```python
from build123d import *

# Parameters (mm, degrees)
BOSS_EXTRUDE1_DEPTH = 6.35
SKETCH2_R           = 3.302
SKETCH2_R_2         = 3.4798
SKETCH2_R_3         = 3.6576
CUT_EXTRUDE1_DEPTH  = 7.35
SHELL5_T            = -2.54
SKETCH5_R           = 6.0198
BOSS_EXTRUDE5_DEPTH = 3.81
SKETCH8_W           = 1.524
SKETCH8_H           = 8.89
CUT_EXTRUDE2_DEPTH  = 6.35
CHAMFER1_SIZE       = 0.635


with BuildPart() as part:
    # Sketch1 → Boss-Extrude1 (new body)
    with BuildSketch(Plane.XY):
        with BuildLine():
            Line((-38.1, 6.35), (38.1, 6.35))
            ThreePointArc((38.1, 6.35), (44.45, 0), (38.1, -6.35))
            Line((38.1, -6.35), (-38.1, -6.35))
            ThreePointArc((-38.1, -6.35), (-44.45, 0), (-38.1, 6.35))
        make_face()
    extrude(amount=BOSS_EXTRUDE1_DEPTH)

    # Sketch2 → Cut-Extrude1 (cut, through all)
    with BuildSketch(Plane.XY.offset(6.35)):
        with Locations((-38.1, 0)):
            Circle(SKETCH2_R)
        with Locations((-12.7, 0)):
            Circle(SKETCH2_R_2)
        with Locations((12.7, 0)):
            Circle(SKETCH2_R_3)
    extrude(amount=-CUT_EXTRUDE1_DEPTH, mode=Mode.SUBTRACT)

    # Shell5
    shell5_openings = [part.faces().sort_by_distance(p)[0] for p in [
        (1.279901808, 0, 6.35),
    ]]
    offset(amount=SHELL5_T, openings=shell5_openings)

    # Sketch5 → Boss-Extrude5 (add)
    with BuildSketch(Plane.XY.offset(2.54)):
        with Locations((38.1, 0)):
            Circle(SKETCH5_R)
    extrude(amount=BOSS_EXTRUDE5_DEPTH)

    # Sketch7 → Revolve1 (revolve)
    with BuildSketch(Plane(origin=(0, 0, 0), x_dir=(1, 0, 0), z_dir=(0, 1, 0))):
        Polygon((35.052, -6.35), (35.052, -12.192), (34.544, -12.7), (34.544, -14.224), (35.56, -15.24), (38.1, -15.24), (38.1, -6.35), align=None)
    revolve(axis=Axis((38.1, 0, 0), (0, 0, 1)))

    # Sketch8 → Cut-Extrude2 (cut, symmetric)
    with BuildSketch(Plane(origin=(0, 0, 0), x_dir=(1, 0, 0), z_dir=(0, 1, 0))):
        with Locations((38.1, -10.795)):
            Rectangle(SKETCH8_W, SKETCH8_H)
    extrude(amount=CUT_EXTRUDE2_DEPTH, both=True, mode=Mode.SUBTRACT)

    # Chamfer1
    chamfer1_edges = [part.edges().sort_by_distance(p)[0] for p in [
        (-41.402, 0, 6.35),
        (-16.1798, 0, 6.35),
        (9.0424, 0, 6.35),
    ]]
    chamfer(chamfer1_edges, length=CHAMFER1_SIZE)


solid = part.part
```
Input: part model. Units: mm. Frame: model coordinates. A direction names the side the tool comes from. Give positions to 0.01 mm unless a question says otherwise; leave off trailing zeros. Order: outer loops, then holes, each group sorted by start corner. A loop starts at its lowest first (then second) coordinate and runs counter-clockwise, first axis right, second up.
1. Pin query (flat end, axial travel): pin 1 Ø4 at (x, y) = (7.5, -2) entering from +Z; pin 2 Ø6 at (x, y) = (12.7, 0) entering from +Z; pin 3 Ø2 at (y, z) = (1.5, 10.5) entering from -X; pin 4 Ø1.5 at (y, z) = (1, 5) entering from +X. Return the tip coordinate at first contact, or that it passes through.
Computed:
pin 1: stops at z = 6.35
pin 2: passes through
pin 3: stops at x = 35.09
pin 4: stops at x = 44.45
2. Draft query along Y for faces 1 (the face through (37.338, 0, 11)), 2 (the face through (0, -3.81, 4)), 3 (the face through (-1, 6.35, 3)). Return one class per face: released by +Y, released by -Y, zero draft, split by the parting line, or undercut.
Computed:
face 1: zero draft
face 2: undercut
face 3: released by +Y
3. Line query: probe 1 along Y at (x, z) = (-19.5, 6); probe 2 along Y at (x, z) = (12.7, 4.3); probe 3 along Y at (x, z) = (-33.5, 6). Output: solid intervals per line, ascending.
Computed:
probe 1: y = -6.35 to -3.81, 3.81 to 6.35
probe 2: y = -6.35 to -3.66, 3.66 to 6.35
probe 3: y = -6.35 to -3.81, -3.6 to 3.6, 3.81 to 6.35
4. Cut plane D-D (y = 0). State how many separate pieces and enclosed holes the cut face has, and give its area (3 significant figures).
Computed:
separate pieces: 4
enclosed holes: 0
area: 321 mm2
5. Cut plane B-B (x = -12.7). Return loops of the section in (y, z) (3 decimals), and give its area (3 significant figures).
Computed:
outline: (-6.35, 0) - (-3.48, 0) - (-3.48, 5.715) - (-4.115, 6.35) - (-6.35, 6.35) - close; (3.48, 0) - (6.35, 0) - (6.35, 6.35) - (4.115, 6.35) - (3.48, 5.715) - close
area: 36.0 mm2
6. Set-up query: faces 4 (the face through (34.908, 0.061, 12.337)), 5 (the face through (41.655, -0.067, 13.473)), 6 (the face through (9.8, -2.23, 2.9)), 7 (the face through (0, 3.81, 4)), 8 (the face through (37, 0, 15.24)). Return all of +Z, -Z, +X, -X, +Y, -Y with unobstructed straight access to the full face (end or side cutting, diameter ignored); none if empty.
Computed:
face 4: -X
face 5: +Z, +X
face 6: +Z, -Z
face 7: +Z
face 8: +Z, +X, -X, +Y, -Y
7. Cut plane A-A (z = 4.5). Return loops of the section in (x, y), and give its area (3 significant figures).
Computed:
outline: (-38.1, -6.35) - (38.1, -6.35) arc R6.35 ccw to (38.1, 6.35) - (-38.1, 6.35) arc R6.35 ccw to start; hole circle Ø6.6 at (-38.1, 0); hole (-33.67, -3.81) - (-17.36, -3.81) arc R6.02 cw to (-17.36, 3.81) - (-33.67, 3.81) arc R5.84 cw to start; hole circle Ø6.96 at (-12.7, 0); hole (-8.04, -3.81) - (7.81, -3.81) arc R6.2 cw to (7.81, 3.81) - (-8.04, 3.81) arc R6.02 cw to start; hole circle Ø7.32 at (12.7, 0); hole (17.59, -3.81) - (33.44, -3.81) arc R6.02 cw to (33.44, 3.81) - (17.59, 3.81) arc R6.2 cw to start
area: 656 mm2
8. Cut plane C-C (z = 8.5). Return loops of the section in (x, y), and give its area (3 significant figures).
Computed:
outline: (37.34, -2.95) - (37.34, 2.95) arc R3.05 ccw to start; (38.86, -2.95) arc R3.05 ccw to (38.86, 2.95) - close
area: 20.0 mm2
